Can you work these out from the model? Positions are in its coordinate system, mm. Give positions to 0.01 mm unless a question says otherwise; leave off trailing zeros. Write each loop counter-clockwise with the first axis right and the second up, starting at its lowest first coordinate (ties: lowest second). Pieces come first, ordered by that corner, then holes.
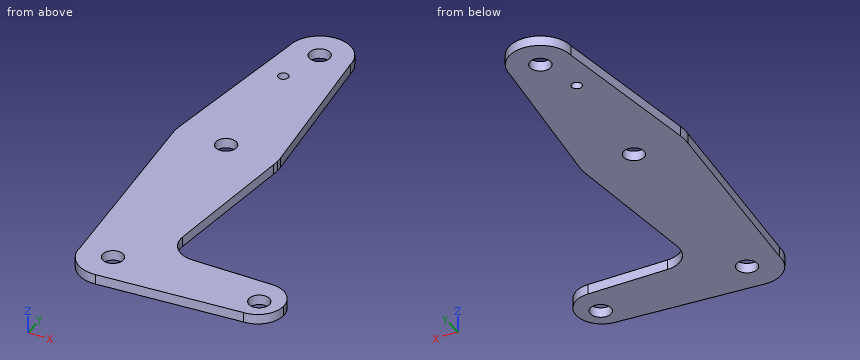
from build123d import *

# Parameters (mm, degrees)
F0_R     = 3.175
F0_R_2   = 1.5875
F1_DEPTH = 3.048


with BuildPart() as f1:
    # F0 (on Top) → F1 (new body)
    with BuildSketch(Plane.XY):
        with BuildLine():
            ThreePointArc((-9.525, 114.3), (0, 104.775), (9.525, 114.3))
            ThreePointArc((9.525, 114.3), (0, 123.825), (-9.525, 114.3))
        make_face()
        with Locations((0, 114.3)):
            Circle(F0_R, mode=Mode.SUBTRACT)
        with BuildLine():
            Line((15.750729, 64.836387), (9.525, 114.3))
            ThreePointArc((9.525, 114.3), (0, 104.775), (-9.525, 114.3))
            Line((-9.525, 114.3), (-15.750729, 64.836387))
            ThreePointArc((-15.750729, 64.836387), (0, 78.728924), (15.750729, 64.836387))
        make_face()
        with Locations((-3.488187, 100.445924)):
            Circle(F0_R_2, mode=Mode.SUBTRACT)
        with BuildLine():
            ThreePointArc((15.875, 62.853924), (15.843902, 63.847101), (15.750729, 64.836387))
            ThreePointArc((15.750729, 64.836387), (0, 78.728924), (-15.750729, 64.836387))
            ThreePointArc((-15.750729, 64.836387), (-15.875, 62.853924), (-15.750729, 60.871462))
            ThreePointArc((-15.750729, 60.871462), (0, 46.978924), (15.750729, 60.871462))
            ThreePointArc((15.750729, 60.871462), (15.843902, 61.860747), (15.875, 62.853924))
        make_face()
        with Locations((-0.282163, 63.186049)):
            Circle(F0_R, mode=Mode.SUBTRACT)
        with BuildLine():
            ThreePointArc((15.750729, 60.871462), (0, 46.978924), (-15.750729, 60.871462))
            Line((-15.750729, 60.871462), (-9.77514, -0.262389))
            ThreePointArc((-9.77514, -0.262389), (-0.044493, 8.829508), (9.265119, -0.693056))
            ThreePointArc((9.265119, -0.693056), (6.725519, -7.168379), (0.460961, -10.190741))
            Line((0.460961, -10.190741), (44.5993, -6.840791))
            ThreePointArc((44.5993, -6.840791), (36.6618, 1.096709), (44.5993, 9.034209))
            Line((44.5993, 9.034209), (19.787523, 9.034209))
            ThreePointArc((19.787523, 9.034209), (13.919598, 11.620349), (11.869256, 17.696266))
            Line((11.869256, 17.696266), (15.750729, 60.871462))
        make_face()
        with BuildLine():
            ThreePointArc((9.265119, -0.693056), (-0.044493, 8.829508), (-9.77514, -0.262389))
            ThreePointArc((-9.77514, -0.262389), (-6.891509, -7.530244), (0.460961, -10.190741))
            ThreePointArc((0.460961, -10.190741), (6.725519, -7.168379), (9.265119, -0.693056))
        make_face()
        with Locations((0.322241, -0.276352)):
            Circle(F0_R, mode=Mode.SUBTRACT)
        with BuildLine():
            ThreePointArc((44.5993, 9.034209), (36.6618, 1.096709), (44.5993, -6.840791))
            ThreePointArc((44.5993, -6.840791), (50.21196, -4.515951), (52.5368, 1.096709))
            ThreePointArc((52.5368, 1.096709), (50.21196, 6.709369), (44.5993, 9.034209))
        make_face()
        with Locations((45.652531, 0.025849)):
            Circle(F0_R, mode=Mode.SUBTRACT)
    extrude(amount=F1_DEPTH)


solid = f1.part
(1) Imagine slicing it at C-C, the plane y = 74. Write out the boundary of the cut face in (x, z), plus the area to 3 significant figures.
Returned:
outline: (-14.6, 0) - (14.6, 0) - (14.6, 3.05) - (-14.6, 3.05) - close
area: 89.0 mm2
(2) Will these pins go through, and if not, where does the flat tip stop? P1, Ø8, axis at x = 19.5, y = 70.5, coming from the -Z side; P2, Ø7.5, axis at x = 45.65, y = 0.03, coming from the -Z side; P3, Ø1, axis at x = 22, z = 2, coming from the -Y side; P4, Ø0.9, axis at x = 26.5, z = 2, coming from the +Y side.
Returned:
P1: passes through
P2: stops at z = 0
P3: stops at y = -8.59
P4: stops at y = 9.03
(3) If I drill on L1, parallel to X at y = 2.5, z = 0.6; L2, parallel to Y at x = -2.5, z = 0.35; L3, parallel to X at y = 40, z = 0.5, over which ranges is the centre line in solid material (lowest first)?
Returned:
L1: x = -10.05 to -1.22, 1.86 to 43.66, 47.64 to 52.41
L2: y = -9.95 to -1.73, 1.18 to 60.91, 65.46 to 99.2, 101.69 to 112.34, 116.26 to 123.49
L3: x = -13.71 to 13.87
(4) Imagine slicing it at A-A, the plane z = 2.4. Give the number of separate pieces and of enclosed holes in the cut face, plus the area to 3 significant figures.
Returned:
separate pieces: 1
enclosed holes: 5
area: 3,840 mm2
(5) Imagine slicing it at B-B, the plane y = 46.5. Write out the boundary of the cut face in (x, z), plus the area to 3 significant figures.
Returned:
outline: (-14.35, 0) - (14.46, 0) - (14.46, 3.05) - (-14.35, 3.05) - close
area: 87.8 mm2
